Model file for the job. Use its own axes, mm. Face numbers are marked on the shaded views. A direction names the side the tool comes from. Round coordinates to 2 decimals unless told otherwise and drop trailing zeros. Loops run counter-clockwise (first coordinate to the right, second up) from the corner with the lowest first, then second, coordinate; pieces in that order, holes last. Notation, with made-up numbers: M -6.5,54.5 L 25.5,54.5 A13 ccw 25.5,58.5 Z; hole C -14,72 d8. An arc over 180 degrees is marked long. Answer in a Markdown table with one row per item.
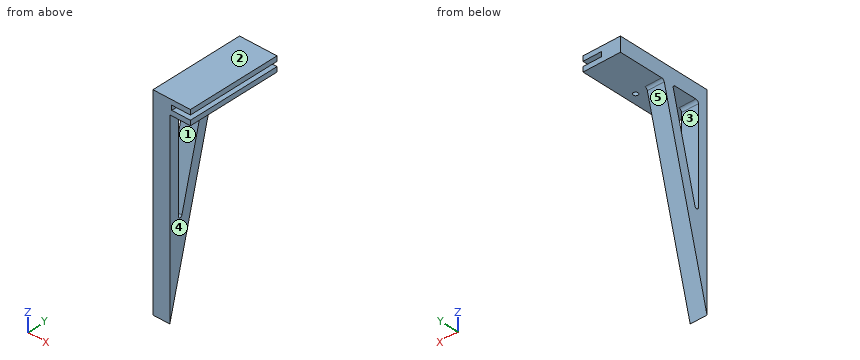
from build123d import *

# Parameters (mm, degrees)
BOSS_EXTRUDE1_DEPTH = 100
EXTRUDE_THIN1_DEPTH = 18
FILLET1_R           = 3
FILLET2_R           = 3
FILLET3_R           = 2
FILLET4_R           = 2
CUT_EXTRUDE1_REACH  = 17.5
SKETCH3_R           = 2.5


with BuildPart() as part:
    # Sketch1 → Boss-Extrude1 (new body)
    with BuildSketch(Plane(origin=(0, 0, 0), x_dir=(1, 0, 0), z_dir=(0, 1, 0))):
        Polygon((0, 0), (20, 0), (20, -5.25), (-20, -5.25), (-20, 10.25), (20, 10.25), (20, 5), (0, 5), align=None)
    extrude(amount=BOSS_EXTRUDE1_DEPTH)

    # Sketch2 → Extrude-Thin1 (add)
    with BuildSketch(Plane.ZY.offset(20)):
        Polygon((-10.25, 0), (-210.25, 0), (-10.25, 50), (-7.82464375, 40.298574999), (-129.018943744, 10), (-10.25, 10), align=None)
    extrude(amount=-EXTRUDE_THIN1_DEPTH)

    # Fillet1
    fillet1_edges = [part.edges().sort_by_distance(p)[0] for p in [
        (-11, 50, -10.25),
    ]]
    fillet(fillet1_edges, radius=FILLET1_R)

    # Fillet2
    fillet2_edges = [part.edges().sort_by_distance(p)[0] for p in [
        (-11, 10, -10.25),
    ]]
    fillet(fillet2_edges, radius=FILLET2_R)

    # Fillet3
    fillet3_edges = [part.edges().sort_by_distance(p)[0] for p in [
        (-11, 39.692235936, -10.25),
    ]]
    fillet(fillet3_edges, radius=FILLET3_R)

    # Fillet4
    fillet4_edges = [part.edges().sort_by_distance(p)[0] for p in [
        (-11, 10, -129.018943744),
    ]]
    fillet(fillet4_edges, radius=FILLET4_R)

    # Sketch3 → Cut-Extrude1 (cut, up to next)
    with BuildSketch(Plane(origin=(0, 0, -10.25), x_dir=(-1, 0, 0), z_dir=(0, 0, -1)), mode=Mode.PRIVATE) as cut_extrude1_sk1:
        with Locations((-10, 50)):
            Circle(SKETCH3_R)
    cut_extrude1_tool1 = extrude(cut_extrude1_sk1.sketch, amount=-CUT_EXTRUDE1_REACH, mode=Mode.PRIVATE) & part.part
    add(cut_extrude1_tool1.solids().sort_by_distance((10, 50, -10.25))[0], mode=Mode.SUBTRACT)


solid = part.part
1. Saw through at C-C (y = 25). Write the cut outline in (x, z), and give its area (3 significant figures).
Verdict:
| item | result |
|---|---|
| outline | M -20,-110.25 L -2,-110.25 L -2,-69.02 L -20,-69.02 Z; M -20,-10.25 L 20,-10.25 L 20,-5 L 0,-5 L 0,0 L 20,0 L 20,5.25 L -20,5.25 Z |
| area | 1,260 mm² |
2. Saw through at A-A (x = 10). Write the cut outline in (y, z), and give its area (3 significant figures).
Verdict:
| item | result |
|---|---|
| outline | M 0,-10.25 L 47.5,-10.25 L 47.5,-5 L 0,-5 Z; M 0,0 L 100,0 L 100,5.25 L 0,5.25 Z; M 52.5,-10.25 L 100,-10.25 L 100,-5 L 52.5,-5 Z |
| area | 1,020 mm² |
3. Wall check: probe 1 along Z at (x, y) = (14, 70); probe 2 along Y at (x, z) = (10, -6); probe 3 along Z at (x, y) = (-5, 95). Give the ranges that are in metal, low to high.
Verdict:
| item | result |
|---|---|
| probe 1 | z = -10.25 to -5, 0 to 5.25 |
| probe 2 | y = 0 to 47.5, 52.5 to 100 |
| probe 3 | z = -10.25 to 5.25 |
4. Pin check, flat tips, straight feed: pin 1 (8 mm diameter, centred on x = 14, y = 60, fed in from -Z); pin 2 (1 mm diameter, centred on y = 23, z = -75.5, fed in from +X); pin 3 (8 mm diameter, centred on x = 1, z = -144.5, fed in from -Y); pin 4 (5.5 mm diameter, centred on x = -6.5, z = -69.5, fed in from +Y) (3 decimals). Stop position of each tip, or through.
Verdict:
| item | result |
|---|---|
| pin 1 | stops at z = -10.25 |
| pin 2 | stops at x = -2 |
| pin 3 | stops at y = 0 |
| pin 4 | stops at y = 35.875 |
5. Saw through at B-B (z = -44). Write the cut outline in (x, y).
Verdict:
| item | result |
|---|---|
| outline | M -20,0 L -2,0 L -2,10 L -20,10 Z; M -20,31.25 L -2,31.25 L -2,41.56 L -20,41.56 Z |
6. Saw through at D-D (x = -9.5). Write the cut outline in (y, z).
Verdict:
| item | result |
|---|---|
| outline | M 0,-210.25 L 49.43,-12.52 A3 cw 52.34,-10.25 L 100,-10.25 L 100,5.25 L 0,5.25 Z; hole M 10,-112.77 A2 ccw 13.94,-113.26 L 39.07,-12.74 A2 ccw 37.13,-10.25 L 13,-10.25 A3 ccw 10,-13.25 Z |
7. Mould opens along Z. For the marked faces 3, 4 and 5 say: +Z half, -Z half, draft (parallel to the pull), parting line (faces both ways), or undercut.
Verdict:
| item | result |
|---|---|
| face 3 | undercut |
| face 4 | draft |
| face 5 | -Z half |
8. Tool access for the marked faces 1 and 2: list every direction of +Z, -Z, +X, -X, +Y, -Y with a clear straight run to the whole face (end or side of a thin tool).
Verdict:
| item | result |
|---|---|
| face 1 | +X, -X |
| face 2 | +Z, +X, -X, +Y, -Y |
